from build123d import *

# Parameters (mm, degrees)
SKETCH1_W           = 12.2
SKETCH1_H           = 45.8
BOSS_EXTRUDE1_DEPTH = 2.5
FILLET1_R           = 6
SKETCH2_W           = 12.2
SKETCH2_H           = 20
BOSS_EXTRUDE2_DEPTH = 2.5
FILLET2_R           = 6
SKETCH3_R           = 1
CUT_EXTRUDE1_DEPTH  = 2.5
CUT_EXTRUDE2_DEPTH  = 2.5
SKETCH5_R           = 2.7
CUT_EXTRUDE3_DEPTH  = 2.5


with BuildPart() as part:
    # Sketch1 → Boss-Extrude1 (new body)
    with BuildSketch(Plane.XY.offset(10)):
        with Locations((-182.131179691, 159.988166791)):
            Rectangle(SKETCH1_W, SKETCH1_H)
    extrude(amount=BOSS_EXTRUDE1_DEPTH)

    # Fillet1
    fillet1_edges = [part.edges().sort_by_distance(p)[0] for p in [
        (-188.231179691, 182.888166791, 11.25),
        (-176.031179691, 182.888166791, 11.25),
        (-176.031179691, 137.088166791, 11.25),
        (-188.231179691, 137.088166791, 11.25),
    ]]
    fillet(fillet1_edges, radius=FILLET1_R)

    # Sketch2 → Boss-Extrude2 (add)
    with BuildSketch(Plane.XY.offset(12.5)):
        with Locations((-182.131179691, 172.965455297)):
            Rectangle(SKETCH2_W, SKETCH2_H)
        with Locations((-182.131179691, 147.010878284)):
            Rectangle(SKETCH2_W, SKETCH2_H)
    extrude(amount=BOSS_EXTRUDE2_DEPTH)

    # Fillet2
    fillet2_edges = [part.edges().sort_by_distance(p)[0] for p in [
        (-176.031179691, 182.965455297, 13.75),
        (-188.231179691, 182.965455297, 13.75),
        (-176.031179691, 137.010878284, 13.75),
        (-188.231179691, 137.010878284, 13.75),
    ]]
    fillet(fillet2_edges, radius=FILLET2_R)

    # Sketch3 → Cut-Extrude1 (cut)
    with BuildSketch(Plane.XY.offset(12.5)):
        with Locations((-185.999682024, 160.057912714)):
            Circle(SKETCH3_R)
        with Locations((-178.054871456, 160.057912714)):
            Circle(SKETCH3_R)
    extrude(amount=-CUT_EXTRUDE1_DEPTH, mode=Mode.SUBTRACT)

    # Sketch4 → Cut-Extrude2 (cut)
    with BuildSketch(Plane.XY.offset(15)):
        with BuildLine():
            Line((-184.138427734, 163.365707397), (-179.861572266, 163.365707397))
            Line((-179.861572266, 163.365707397), (-178.824890137, 177.264755249))
            ThreePointArc((-178.824890137, 177.264755249), (-182, 180.059517658), (-185.175109863, 177.264755249))
            Line((-185.175109863, 177.264755249), (-184.138427734, 163.365707397))
        make_face()
        with BuildLine():
            Line((-184.138427734, 156.610626184), (-185.175109863, 142.711578332))
            ThreePointArc((-185.175109863, 142.711578332), (-182, 139.916815923), (-178.824890137, 142.711578332))
            Line((-178.824890137, 142.711578332), (-179.861572266, 156.610626184))
            Line((-179.861572266, 156.610626184), (-184.138427734, 156.610626184))
        make_face()
    extrude(amount=-CUT_EXTRUDE2_DEPTH, mode=Mode.SUBTRACT)

    # Sketch5 → Cut-Extrude3 (cut)
    with BuildSketch(Plane.XY.offset(12.5)):
        with Locations((-182.080577922, 176.90016829)):
            Circle(SKETCH5_R)
        with Locations(Location((-182.080577922, 143.076165291, 0), (0, 0, 180))):
            Circle(SKETCH5_R)
    extrude(amount=-CUT_EXTRUDE3_DEPTH, mode=Mode.SUBTRACT)


solid = part.part
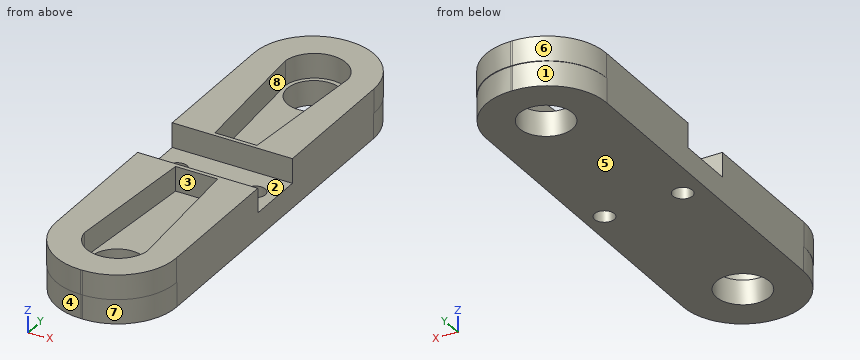
Geometry check sheet. Reference: the model listing, model coordinates, mm. Face numbers are marked on the shaded views. A direction names the side the tool comes from. Give positions to 0.01 mm unless a question says otherwise; leave off trailing zeros. Write each loop counter-clockwise with the first axis right and the second up, starting at its lowest first coordinate (ties: lowest second). Pieces come first, ordered by that corner, then holes.
1) Cross-section at C-C (x = -186). Record the boundary of the cut face in (y, z).
Values follow:
outline: (138.34, 12.5) - (138.42, 12.5) - (138.42, 10) - (159.06, 10) - (159.06, 12.5) - (157.01, 12.5) - (157.01, 15) - (138.34, 15) - close; (161.06, 10) - (181.56, 10) - (181.56, 12.5) - (181.63, 12.5) - (181.63, 15) - (162.97, 15) - (162.97, 12.5) - (161.06, 12.5) - close
2) Cross-section at D-D (y = 159.5). Record the boundary of the cut face in (x, z), plus the area to 3 significant figures.
Values follow:
outline: (-188.23, 10) - (-186.83, 10) - (-186.83, 12.5) - (-188.23, 12.5) - close; (-185.17, 10) - (-178.88, 10) - (-178.88, 12.5) - (-185.17, 12.5) - close; (-177.22, 10) - (-176.03, 10) - (-176.03, 12.5) - (-177.22, 12.5) - close
area: 22.2 mm2
3) Set-up check for the marked faces 1, 2, 3 and 4: record each of +Z, -Z, +X, -X, +Y, -Y from which the full face is reachable in a straight line by a thin tool's end or side.
Values follow:
face 1: -Z, -X, +Y
face 2: +Z, +X, -X
face 3: +Z
face 4: -Z, -X, -Y
4) Cross-section at A-A (z = 13.5). Record the boundary of the cut face in (x, y), plus the area to 3 significant figures.
Values follow:
outline: (-188.23, 143.01) arc R6 ccw to (-182.23, 137.01) - (-182.03, 137.01) arc R6 ccw to (-176.03, 143.01) - (-176.03, 157.01) - (-188.23, 157.01) - close; (-188.23, 162.97) - (-176.03, 162.97) - (-176.03, 176.97) arc R6 ccw to (-182.03, 182.97) - (-182.23, 182.97) arc R6 ccw to (-188.23, 176.97) - close; hole (-185.18, 142.71) arc R3.2 ccw to (-178.82, 142.71) - (-179.86, 156.61) - (-184.14, 156.61) - close; hole (-185.18, 177.26) - (-184.14, 163.37) - (-179.86, 163.37) - (-178.82, 177.26) arc R3.2 ccw to start
area: 282 mm2
5) Go/stop test with flat-tipped pins: pin 1 Ø3 at (x, y) = (-181, 175.5) entering from +Z; pin 2 Ø0.8 at (x, z) = (-180, 13.5) entering from -Y. Record where each tip stops, or that it passes through.
Values follow:
pin 1: stops at z = 12.5
pin 2: stops at y = 137.24
6) Release check for a two-part mould opening along X. For the marked faces 5, 6, 7 and 8 record: released by +X, released by -X, zero draft, split by the parting line, or undercut.
Values follow:
face 5: zero draft
face 6: released by -X
face 7: released by +X
face 8: undercut
7) Thickness scan on line 1 (Y direction, x = -181, z = 13.25); line 2 (Y direction, x = -183.25, z = 14.1); line 3 (X direction, y = 177, z = 11.4). Record the ranges inside material, lowest first.
Values follow:
line 1: y = 137.1 to 140.08, 156.61 to 157.01, 162.97 to 163.37, 179.9 to 182.88
line 2: y = 137.1 to 140.17, 156.61 to 157.01, 162.97 to 163.37, 179.81 to 182.88
line 3: x = -188.23 to -184.78, -179.38 to -176.03
